from build123d import *

# Parameters (mm, degrees)
F0_W     = 504.825
F0_H     = 244.475
F1_DEPTH = 19.05
F4_DEPTH = 19.05
F5_DEPTH = 19.05
F6_R     = 1.984375
F7_DEPTH = 19.05


with BuildPart() as f1:
    # F0 (on Right) → F1 (new body)
    with BuildSketch(Plane.YZ):
        Rectangle(F0_W, F0_H)
    extrude(amount=F1_DEPTH)

    # F3 (on face) → F4 (cut)
    with BuildSketch(Plane(origin=(0, 252.4125, 0), x_dir=(-1, 0, 0), z_dir=(0, 1, 0))):
        with BuildLine():
            Line((0, 77.7875), (0, 122.2375))
            Line((0, 122.2375), (-19.05, 122.2375))
            Line((-19.05, 122.2375), (-19.05, 65.761152))
            ThreePointArc((-19.05, 65.761152), (-18.038918, 69.19895), (-15.327651, 71.541978))
            Line((-15.327651, 71.541978), (-2.839702, 77.218326))
            ThreePointArc((-2.839702, 77.218326), (-1.556345, 77.643575), (-0.21205, 77.7875))
            Line((-0.21205, 77.7875), (0, 77.7875))
        make_face()
        with BuildLine():
            Line((0, -26.9875), (0, 26.9875))
            Line((0, 26.9875), (-0.21205, 26.9875))
            ThreePointArc((-0.21205, 26.9875), (-1.556345, 27.131425), (-2.839702, 27.556674))
            Line((-2.839702, 27.556674), (-15.327651, 33.233022))
            ThreePointArc((-15.327651, 33.233022), (-18.038918, 35.57605), (-19.05, 39.013848))
            Line((-19.05, 39.013848), (-19.05, -39.013848))
            ThreePointArc((-19.05, -39.013848), (-18.038918, -35.57605), (-15.327651, -33.233022))
            Line((-15.327651, -33.233022), (-2.839702, -27.556674))
            ThreePointArc((-2.839702, -27.556674), (-1.556345, -27.131425), (-0.21205, -26.9875))
            Line((-0.21205, -26.9875), (0, -26.9875))
        make_face()
        with BuildLine():
            Line((0, -122.2375), (0, -77.7875))
            Line((0, -77.7875), (-0.21205, -77.7875))
            ThreePointArc((-0.21205, -77.7875), (-1.556345, -77.643575), (-2.839702, -77.218326))
            Line((-2.839702, -77.218326), (-15.327651, -71.541978))
            ThreePointArc((-15.327651, -71.541978), (-18.038918, -69.19895), (-19.05, -65.761152))
            Line((-19.05, -65.761152), (-19.05, -122.2375))
            Line((-19.05, -122.2375), (0, -122.2375))
        make_face()
    extrude(amount=-F4_DEPTH, mode=Mode.SUBTRACT)

    # F2 (on face) → F5 (cut)
    with BuildSketch(Plane.XZ.offset(252.4125)):
        with BuildLine():
            Line((0, 122.2375), (0, 77.7875))
            Line((0, 77.7875), (0.21205, 77.7875))
            ThreePointArc((0.21205, 77.7875), (1.556345, 77.643575), (2.839702, 77.218326))
            Line((2.839702, 77.218326), (15.327651, 71.541978))
            ThreePointArc((15.327651, 71.541978), (18.038918, 69.19895), (19.05, 65.761152))
            Line((19.05, 65.761152), (19.05, 122.2375))
            Line((19.05, 122.2375), (0, 122.2375))
        make_face()
        with BuildLine():
            Line((0, 26.9875), (0, -26.9875))
            Line((0, -26.9875), (0.21205, -26.9875))
            ThreePointArc((0.21205, -26.9875), (1.556345, -27.131425), (2.839702, -27.556674))
            Line((2.839702, -27.556674), (15.327651, -33.233022))
            ThreePointArc((15.327651, -33.233022), (18.038918, -35.57605), (19.05, -39.013848))
            Line((19.05, -39.013848), (19.05, 39.013848))
            ThreePointArc((19.05, 39.013848), (18.038918, 35.57605), (15.327651, 33.233022))
            Line((15.327651, 33.233022), (2.839702, 27.556674))
            ThreePointArc((2.839702, 27.556674), (1.556345, 27.131425), (0.21205, 26.9875))
            Line((0.21205, 26.9875), (0, 26.9875))
        make_face()
        with BuildLine():
            Line((0, -77.7875), (0, -122.2375))
            Line((0, -122.2375), (19.05, -122.2375))
            Line((19.05, -122.2375), (19.05, -65.761152))
            ThreePointArc((19.05, -65.761152), (18.038918, -69.19895), (15.327651, -71.541978))
            Line((15.327651, -71.541978), (2.839702, -77.218326))
            ThreePointArc((2.839702, -77.218326), (1.556345, -77.643575), (0.21205, -77.7875))
            Line((0.21205, -77.7875), (0, -77.7875))
        make_face()
    extrude(amount=-F5_DEPTH, mode=Mode.SUBTRACT)

    # F6 (on face) → F7 (cut)
    with BuildSketch(Plane(origin=(0, 0, 0), x_dir=(0, -1, 0), z_dir=(-1, 0, 0))):
        with Locations((-242.8875, -52.3875)):
            Circle(F6_R)
        with Locations((-242.8875, 52.3875)):
            Circle(F6_R)
        with Locations((242.8875, 52.3875)):
            Circle(F6_R)
        with Locations((242.8875, -52.3875)):
            Circle(F6_R)
    extrude(amount=-F7_DEPTH, mode=Mode.SUBTRACT)


solid = f1.part
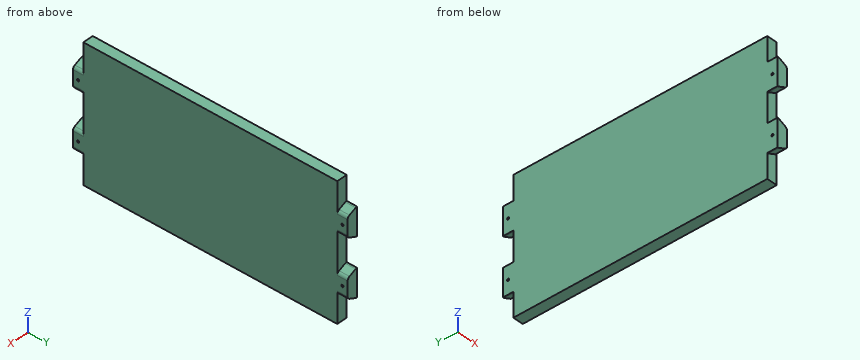
Read the model definition and answer for the solid it produces. Units are mm, in the model's axes. Give positions to 0.01 mm unless a question says otherwise; leave off trailing zeros. Write each loop counter-clockwise with the first axis right and the second up, starting at its lowest first coordinate (ties: lowest second). Pieces come first, ordered by that corner, then holes. Notation, with made-up numbers: (-3.5, 28) - (42.5, 28) arc R17 cw to (42.5, 47) - close; hole circle Ø6 at (88.5, -12). An arc over 180 degrees is marked (long way). Use CSV: the item, a comma, the result in double quotes. Start each with the question number.
Item 1: The part is cut by section B-B, the plane z = -86. Give the vertices of the cut face in (x, y), and give its area (3 significant figures).
Item 2: Flat-ended cylindrical pins translate along their axes: P1, Ø5.5, axis at x = 9.5, z = 96.5, coming from the -Y side; P2, Ø4, axis at x = 14, z = -11.5, coming from the +Y side. Find the tip coordinate at first contact, or state that the pin passes through.
Item 3: The part is cut by section A-A, the plane x = 6.25. Give the vertices of the cut face in (y, z), and give its area (3 significant figures).
Item 4: Consider line 1 (Y direction, x = 12.5, z = 2.5). Determine where the line is inside the solid, lowest interval first.
Taken from the geometry:
1,outline,"(0, -233.36) - (19.05, -233.36) - (19.05, 233.36) - (0, 233.36) - close"
1,area,"8,890 mm2"
2,P1,"y = -233.36"
2,P2,"y = 233.36"
3,outline,"(-252.41, -75.67) - (-233.36, -75.67) - (-233.36, -122.24) - (233.36, -122.24) - (233.36, -75.67) - (252.41, -75.67) - (252.41, -29.11) - (233.36, -29.11) - (233.36, 29.11) - (252.41, 29.11) - (252.41, 75.67) - (233.36, 75.67) - (233.36, 122.24) - (-233.36, 122.24) - (-233.36, 75.67) - (-252.41, 75.67) - (-252.41, 29.11) - (-233.36, 29.11) - (-233.36, -29.11) - (-252.41, -29.11) - close; hole circle Ø3.97 at (-242.89, -52.39); hole circle Ø3.97 at (-242.89, 52.39); hole circle Ø3.97 at (242.89, -52.39); hole circle Ø3.97 at (242.89, 52.39)"
3,area,"118,000 mm2"
4,line 1,"-233.36 to 233.36"
